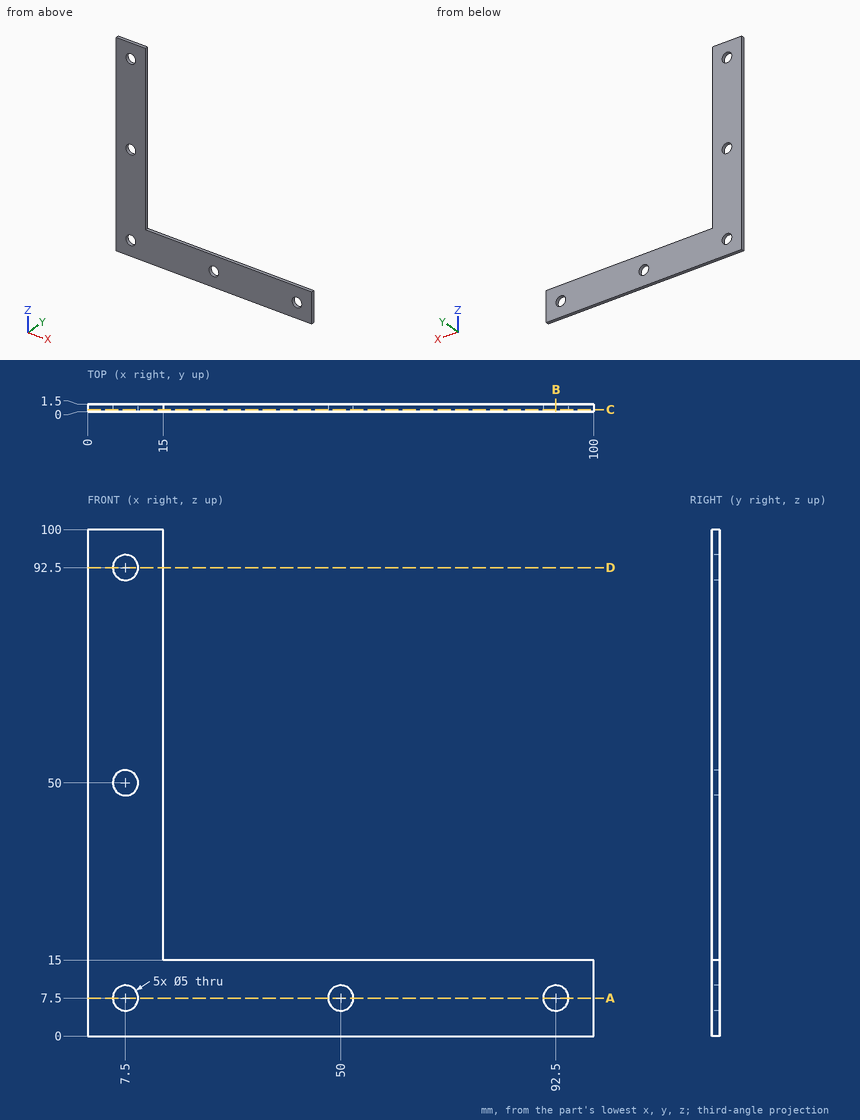
Answer from the drawing. Dimensions are ordinates in mm from the lowest x, y and z of the part. Give positions to 0.01 mm unless a question says otherwise; leave off trailing zeros. Order: outer loops, then holes, each group sorted by start corner. A loop starts at its lowest first (then second) coordinate and runs counter-clockwise, first axis right, second up. Notation, with made-up numbers: (-23, 78) -> (-8, 78) arc R19 cw to (-8, 85) -> close; hole circle Ø11 at (-1.5, 78.5). An arc over 180 degrees is marked (long way). Answer as a JSON object with one key per item and string values. Group by question number.
1. Consider line 1 along Z through (x, y) = (7.5, 0.6); line 2 along Z through (x, y) = (92.5, 1.1); line 3 along X through (y, z) = (1.2, 8.5). Determine where each line is inside the solid, lowest interval first. Write a range as [from, to].
2. Section B-B on x = 92.5 is taken. Determine the outline of the cut face in (y, z).
3. Section D-D on z = 92.5 is taken. Determine the outline of the cut face in (x, y).
4. Section A-A on z = 7.5 is taken. Determine the outline of the cut face in (x, y), plus the area to 4 significant figures.
5. Section C-C on y = 0.4 is taken. Determine the outline of the cut face in (x, z).
Result sheet:
{
 "1": {"line 1": "z = [0, 5], [10, 47.5], [52.5, 90], [95, 100]", "line 2": "z = [0, 5], [10, 15]", "line 3": "x = [0, 5.21], [9.79, 47.71], [52.29, 90.21], [94.79, 100]"},
 "2": {"outline": "(0, 0) -> (1.5, 0) -> (1.5, 5) -> (0, 5) -> close; (0, 10) -> (1.5, 10) -> (1.5, 15) -> (0, 15) -> close"},
 "3": {"outline": "(0, 0) -> (5, 0) -> (5, 1.5) -> (0, 1.5) -> close; (10, 0) -> (15, 0) -> (15, 1.5) -> (10, 1.5) -> close"},
 "4": {"outline": "(0, 0) -> (5, 0) -> (5, 1.5) -> (0, 1.5) -> close; (10, 0) -> (47.5, 0) -> (47.5, 1.5) -> (10, 1.5) -> close; (52.5, 0) -> (90, 0) -> (90, 1.5) -> (52.5, 1.5) -> close; (95, 0) -> (100, 0) -> (100, 1.5) -> (95, 1.5) -> close", "area": "127.5 mm^2"},
 "5": {"outline": "(0, 0) -> (100, 0) -> (100, 15) -> (15, 15) -> (15, 100) -> (0, 100) -> close; hole circle Ø5 at (7.5, 7.5); hole circle Ø5 at (7.5, 50); hole circle Ø5 at (7.5, 92.5); hole circle Ø5 at (50, 7.5); hole circle Ø5 at (92.5, 7.5)"}
}
